Here's the drawing with two shaded views (mm, measured from the low corner). I have some questions. A direction names the side the tool comes from. Coordinates: 2 decimals unless noted, no trailing zeros. Write each loop counter-clockwise with the first axis right and the second up, starting at its lowest first coordinate (ties: lowest second). Pieces come first, ordered by that corner, then holes. Notation, with made-up numbers: M -28,34 L -18,34 A29 cw -18,64 Z; hole C 11,24 d3. An arc over 180 degrees is marked long. Use one line per item in the form item = value. Start each with the question number.
1. Please list where these lines run through material, in increasing order: line 1 along Y through (x, z) = (8.75, 0.4); line 2 along X through (y, z) = (4.5, 1.65). Write a range as [from, to].
2. I want a section at B-B, the plane x = 9.25. List the corners of the cut face in (y, z) for me, plus the area to 4 significant figures.
3. I want a section at A-A, the plane z = 0.2. List the corners of the cut face in (x, y) for me, plus the area to 4 significant figures.
4. Thinking about a two-plate mould opening in Y: for the marked faces 3, 4 and 5, which applies, released by +Y, released by -Y, zero draft, split by the parting line, or undercut?
5. On a 3-axis mill with a long thin cutter (end or side, diameter ignored), from which of +Z, -Z, +X, -X, +Y, -Y can I reach the whole of each face in a straight line? I mean the marked faces 1 and 2. Say none if no direction works.
6. I'm going to push a flat-ended pin straight in: pin 1 Ø1.2 at (y, z) = (4, 1) entering from +X. Where does the tip first touch, or does it pass through?
7. I want a section at C-C, the plane y = 5. List the corners of the cut face in (x, z) for me, plus the area to 3 significant figures.
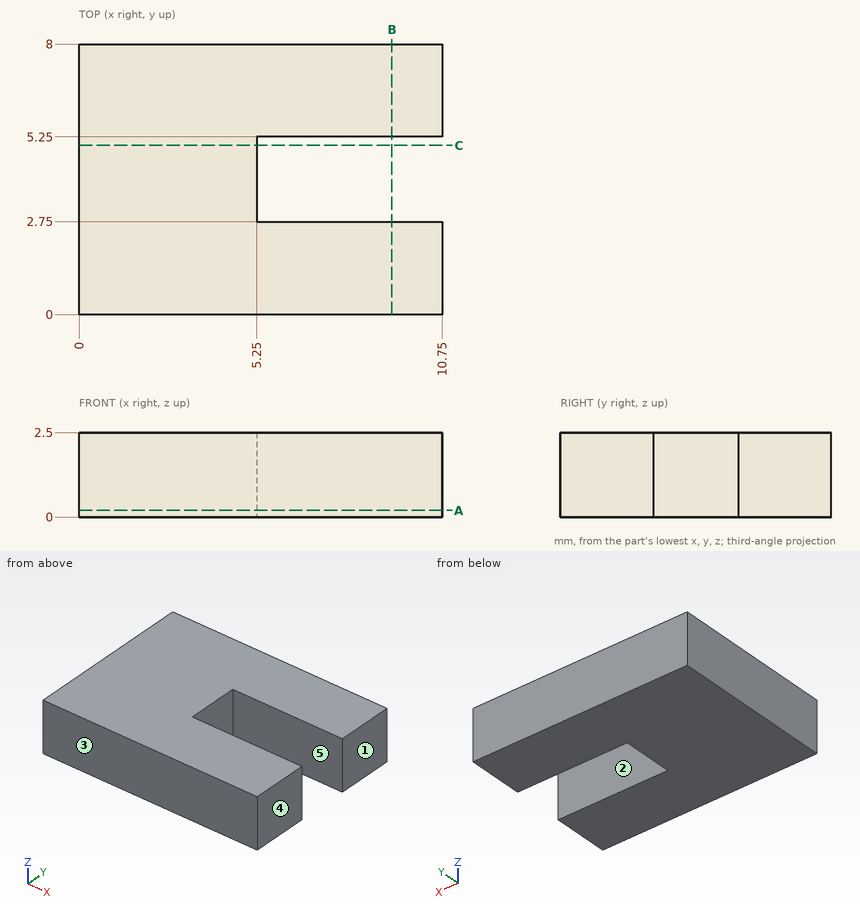
Answer list:
q1.line_1 = [0, 2.75], [5.25, 8]
q1.line_2 = [0, 5.25]
q2.outline = M 0,0 L 2.75,0 L 2.75,2.5 L 0,2.5 Z; M 5.25,0 L 8,0 L 8,2.5 L 5.25,2.5 Z
q2.area = 13.75 mm²
q3.outline = M 0,0 L 10.75,0 L 10.75,2.75 L 5.25,2.75 L 5.25,5.25 L 10.75,5.25 L 10.75,8 L 0,8 Z
q3.area = 72.25 mm²
q4.face_3 = released by -Y
q4.face_4 = zero draft
q4.face_5 = undercut
q5.face_1 = +Z, -Z, +X, +Y, -Y
q5.face_2 = +Z, -Z, +X
q6.pin_1 = 5.25
q7.outline = M 0,0 L 5.25,0 L 5.25,2.5 L 0,2.5 Z
q7.area = 13.1 mm²
